Design review of the part built by this model. Coordinates are the model's own, in mm. Face numbers are marked on the shaded views. A direction names the side the tool comes from. Give positions to 0.01 mm unless a question says otherwise; leave off trailing zeros. Order: outer loops, then holes, each group sorted by start corner. A loop starts at its lowest first (then second) coordinate and runs counter-clockwise, first axis right, second up. Notation, with made-up numbers: (-40, 89) -> (-32, 89) arc R26 cw to (-32, 118) -> close; hole circle Ø5 at (65, 3). An arc over 180 degrees is marked (long way). Return JSON: item names as keys, results as strings.
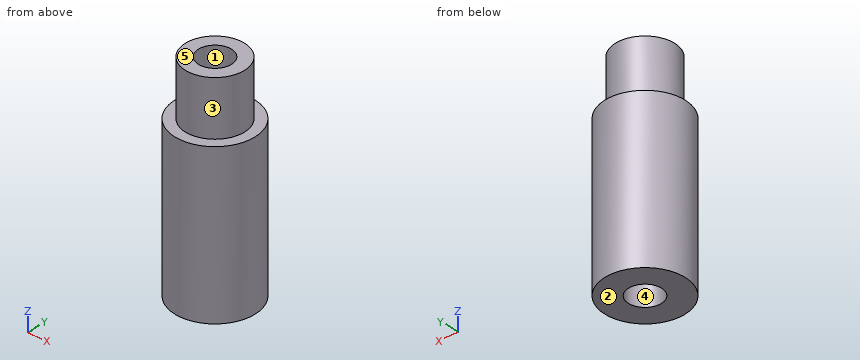
```python
from build123d import *

# Parameters (mm, degrees)
SKETCH_1_R               = 4
EXTRUDE_1_DEPTH          = 7.9
SKETCH_2_R               = 2.95
EXTRUDE_2_DEPTH          = 5.5
M4X0_7_1_D               = 3.3
M4X0_7_1_DEPTH           = 7
M4X0_7_1_TIP             = 0.991420021
M4X0_7_1_ON_FACE_2_D     = 3.3
M4X0_7_1_ON_FACE_2_DEPTH = 7
M4X0_7_1_ON_FACE_2_TIP   = 0.991420021


with BuildPart() as part:
    # ｽｹｯﾁ1 → ﾎﾞｽ - 押し出し1 (new body, symmetric)
    with BuildSketch(Plane.XY):
        Circle(SKETCH_1_R)
    extrude(amount=EXTRUDE_1_DEPTH, both=True)

    # ｽｹｯﾁ2 → ﾎﾞｽ - 押し出し2 (add)
    with BuildSketch(Plane.XY.offset(7.9)):
        Circle(SKETCH_2_R)
    extrude(amount=EXTRUDE_2_DEPTH)

    # M4x0.7 ねじ穴1
    with Locations(Plane(origin=(0, 0, -7.9), x_dir=(-1, 0, 0), z_dir=(0, 0, -1))):
        with Locations((0, 0)):
            Hole(M4X0_7_1_D / 2, depth=M4X0_7_1_DEPTH)
            with Locations((0, 0, -(M4X0_7_1_DEPTH + M4X0_7_1_TIP / 2))):  # 118° drill point
                Cone(0, M4X0_7_1_D / 2, M4X0_7_1_TIP, mode=Mode.SUBTRACT)

    # M4x0.7 ねじ穴1 on face 2
    with Locations(Plane.XY.offset(13.4)):
        with Locations((0, 0)):
            Hole(M4X0_7_1_ON_FACE_2_D / 2, depth=M4X0_7_1_ON_FACE_2_DEPTH)
            with Locations((0, 0, -(M4X0_7_1_ON_FACE_2_DEPTH + M4X0_7_1_ON_FACE_2_TIP / 2))):  # 118° drill point
                Cone(0, M4X0_7_1_ON_FACE_2_D / 2, M4X0_7_1_ON_FACE_2_TIP, mode=Mode.SUBTRACT)


solid = part.part
```
Item 1: Machinability: for the marked faces 4 and 5, which of the approach directions +Z, -Z, +X, -X, +Y, -Y give a long, thin tool a straight path to every point of the face, cutting with its end or side? Answer none if there is none.
Result set:
{"face 4": "-Z", "face 5": "+Z, +X, -X, +Y, -Y"}
Item 2: Add section C-C (y = 3.75). Give the boundary of the cut face in (x, z).
Result set:
{"outline": "(-1.39, -7.9) -> (1.39, -7.9) -> (1.39, 7.9) -> (-1.39, 7.9) -> close"}
Item 3: Add section B-B (z = 2). Give the boundary of the cut face in (x, y), plus the area to 3 significant figures.
Result set:
{"outline": "circle Ø8 at (0, 0)", "area": "50.3 mm^2"}
Item 4: Add section A-A (z = 10). Give the boundary of the cut face in (x, y).
Result set:
{"outline": "circle Ø5.9 at (0, 0); hole circle Ø3.3 at (0, 0)"}
Item 5: Wall thickness on L1, parallel to Y at x = 0, z = 10.75; L2, parallel to Y at x = 0, z = -4; L3, parallel to Z at x = -2, y = -3.25: over which ranges is each line inside the solid? List them lowest first. Write a range as [from, to].
Result set:
{"L1": "y = [-2.95, -1.65], [1.65, 2.95]", "L2": "y = [-4, -1.65], [1.65, 4]", "L3": "z = [-7.9, 7.9]"}
Item 6: Mouldability with a two-part tool opening along X and no side actions: class the marked faces 1, 2 and 3 as released by +X, released by -X, zero draft, split by the parting line, or undercut.
Result set:
{"face 1": "undercut", "face 2": "zero draft", "face 3": "split by the parting line"}
Item 7: Add section D-D (x = 3.25). Give the boundary of the cut face in (y, z), plus the area to 3 significant figures.
Result set:
{"outline": "(-2.33, -7.9) -> (2.33, -7.9) -> (2.33, 7.9) -> (-2.33, 7.9) -> close", "area": "73.7 mm^2"}
Item 8: For pin 1 (2 mm diameter, centred on x = 2, z = 9, fed in from -Y); pin 2 (1 mm diameter, centred on x = 1, z = 0, fed in from -Y), all flat-tipped, find the tip position at first contact; note any pin that passes through.
Result set:
{"pin 1": "stops at y = -2.78", "pin 2": "stops at y = -3.97"}
